Part model, mm, in its own coordinate system. A direction names the side the tool comes from. Round coordinates to 2 decimals unless told otherwise and drop trailing zeros. Write each loop counter-clockwise with the first axis right and the second up, starting at its lowest first coordinate (ties: lowest second). Pieces come first, ordered by that corner, then holes.
Autodesk Inventor part; units mm, degrees
ref_plane "YZ Plane" through (0, 0, 0) normal (1, 0, 0) x (0, 1, 0)
ref_plane "XZ Plane" through (0, 0, 0) normal (0, 1, 0) x (-1, 0, 0)
ref_plane "XY Plane" through (0, 0, 0) normal (0, 0, 1) x (1, 0, 0)
sketch "Sketch1" plane through (0, 0, 0) normal (0, 0, 1) x (1, 0, 0)
  line L0 (0, 0) -> (25.4, 0)
  line L1 (25.4, 0) -> (25.4, 25.4)
  line L2 (25.4, 25.4) -> (0, 25.4)
  line L3 (0, 25.4) -> (0, 0)
  circle A0 centre (6.35, 19.05) radius 2.4892
  line L4 (12.7, 25.4) -> (12.7, 0) construction
  line L5 (0, 12.7) -> (25.4, 12.7) construction
  circle A1 centre (19.05, 19.05) radius 2.4892
  circle A2 centre (6.35, 6.35) radius 2.4892
  circle A3 centre (19.05, 6.35) radius 2.4892
  dimension "d0" = 25.4
  dimension "d1" = 25.4
  dimension "d2" = 4.9784
  dimension "d3" = 6.35
  dimension "d4" = 6.35
extrude "Extrusion1" add sketch "Sketch1" along normal blind 1.5875
sketch "Sketch2" plane through (0, 0, 0) normal (-1, 0, 0) x (0, 0, 1)
  line L0 (0, 25.4) -> (0, 0)
  line L1 (0, 0) -> (1.5875, 0)
  line L2 (0, 25.4) -> (1.5875, 25.4)
  line L3 (1.5875, 25.4) -> (26.9875, 0)
  line L4 (1.5875, 25.4) -> (37.5085, 25.4) construction
  line L5 (26.9875, 0) -> (1.5875, 0)
  line L6 (1.5875, 25.4) -> (1.5875, 0)
  dimension "d7" = 45
extrude "Extrusion2" add sketch "Sketch2" along normal blind 1.5875
ref_plane "Work Plane1" through (12.7, 0, 0) normal (1, 0, 0) x (0, 0, -1)
mirror "Mirror1" about plane through (12.7, 0, 0) normal (1, 0, 0) of "Extrusion2"
sketch "Sketch3" plane through (0, 0, 1.5875) normal (0, -1, 0) x (1, 0, 0)
  line L0 (-1.5875, 25.4) -> (26.9875, 25.4)
  line L1 (26.9875, 25.4) -> (26.9875, -1.5875)
  line L2 (26.9875, -1.5875) -> (-1.5875, -1.5875)
  line L3 (-1.5875, -1.5875) -> (-1.5875, 25.4)
  point P0 (0, -1.5875)
extrude "Extrusion3" add sketch "Sketch3" along normal blind 1.5875
equation "\"d4\" = d3"
properties part number "Milled Flange Support" material "Aluminum 6061"
Q1. Wall check: L1, parallel to Y at x = 6.35, z = 1; L2, parallel to X at y = 0.5, z = 17.5; L3, parallel to Z at x = 23, y = 9.25. Give the ranges that are in metal, low to high.
Values follow:
L1: y = -1.59 to 3.86, 8.84 to 16.56, 21.54 to 25.4
L2: x = -1.59 to 0, 25.4 to 26.99
L3: z = 0 to 1.59
Q2. Which spindle directions (+Z, -Z, +X, -X, +Y, -Y) get a long thin tool onto all of the face, cutting with end or side? Do faces 5 (the flat face through (-1.588, 9, 10)), 6 (the flat face through (13, 0, 14)). Say none if no direction does.
Values follow:
face 5: +Z, -Z, -X, +Y, -Y
face 6: +Z, +Y
Q3. Cut at B-B on y = 20. Write the cut outline in (x, z).
Values follow:
outline: (-1.59, 0) - (4.05, 0) - (4.05, 1.59) - (0, 1.59) - (0, 6.99) - (-1.59, 6.99) - close; (8.65, 0) - (16.75, 0) - (16.75, 1.59) - (8.65, 1.59) - close; (21.35, 0) - (26.99, 0) - (26.99, 6.99) - (25.4, 6.99) - (25.4, 1.59) - (21.35, 1.59) - close
Q4. Cut at D-D on x = 19.25. Write the cut outline in (y, z), plus the area to 3 significant figures.
Values follow:
outline: (-1.59, 0) - (3.87, 0) - (3.87, 1.59) - (0, 1.59) - (0, 26.99) - (-1.59, 26.99) - close; (8.83, 0) - (16.57, 0) - (16.57, 1.59) - (8.83, 1.59) - close; (21.53, 0) - (25.4, 0) - (25.4, 1.59) - (21.53, 1.59) - close
area: 67.4 mm2
Q5. Cut at C-C on z = 4.5. Write the cut outline in (x, y).
Values follow:
outline: (-1.59, -1.59) - (26.99, -1.59) - (26.99, 22.49) - (25.4, 22.49) - (25.4, 0) - (0, 0) - (0, 22.49) - (-1.59, 22.49) - close
Q6. Cut at A-A on x = 6.35. Write the cut outline in (y, z), plus the area to 3 significant figures.
Values follow:
outline: (-1.59, 0) - (3.86, 0) - (3.86, 1.59) - (0, 1.59) - (0, 26.99) - (-1.59, 26.99) - close; (8.84, 0) - (16.56, 0) - (16.56, 1.59) - (8.84, 1.59) - close; (21.54, 0) - (25.4, 0) - (25.4, 1.59) - (21.54, 1.59) - close
area: 67.4 mm2
Q7. Drop flat-ended pins along their axis: pin 1 (4 mm diameter, centred on x = 17, y = 17, fed in from +Z); pin 2 (6.5 mm diameter, centred on x = 6.35, y = 6.35, fed in from -Z); pin 3 (12.5 mm diameter, centred on x = 17, z = 11, fed in from +Y); pin 4 (4 mm diameter, centred on x = 19.05, y = 19.05, fed in from -Z). Give the stop position or say it passes through.
Values follow:
pin 1: stops at z = 1.59
pin 2: stops at z = 0
pin 3: stops at y = 0
pin 4: passes through
Q8. Mould opens along X. For faces 1 (the cylindrical face through (16.563, 6.241, 0.783)), 2 (the flat face through (13, 13, 1.588)), 3 (the flat face through (13, 25.4, 1)), 4 (the flat face through (26.988, 9, 11)) say: +X half, -X half, draft (parallel to the pull), parting line (faces both ways), or undercut.
Values follow:
face 1: undercut
face 2: undercut
face 3: draft
face 4: +X half
